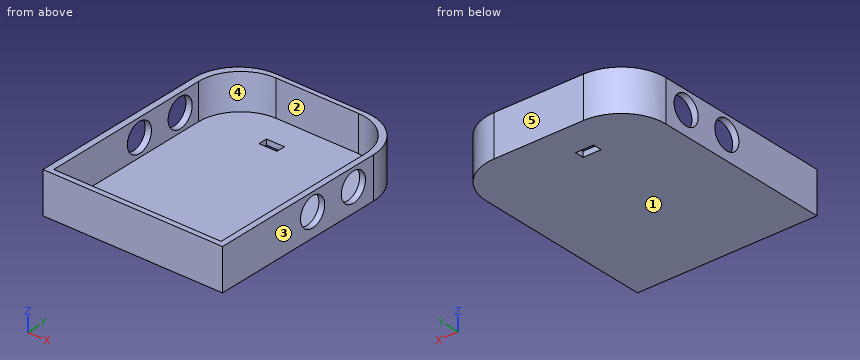
```python
from build123d import *

# Parameters (mm, degrees)
BOX008_W        = 10
BOX008_H        = 5
BOX008_DEPTH    = 10
PAD_DEPTH       = 23
POCKET_DEPTH    = 20
SKETCH002_R     = 8
POCKET001_DEPTH = 100.001


with BuildPart() as cube008:
    # Box008 → Box008 (new body)
    with BuildSketch(Plane(origin=(-15, 40, -4), x_dir=(1, 0, 0), z_dir=(0, 0, 1))):
        with Locations((5, 2.5)):
            Rectangle(BOX008_W, BOX008_H)
    extrude(amount=BOX008_DEPTH)


with BuildPart() as cut012:
    # Sketch → Pad (new body)
    with BuildSketch(Plane.XY):
        with BuildLine():
            Line((-50, 38.45712), (-50, -61.54288))
            Line((-50, -61.54288), (50, -61.54288))
            Line((50, -61.54288), (50, 38.45712))
            ThreePointArc((50, 38.45712), (42.67767, 56.13479), (25, 63.45712))
            Line((25, 63.45712), (-25, 63.45712))
            ThreePointArc((-25, 63.45712), (-42.67767, 56.13479), (-50, 38.45712))
        make_face()
    extrude(amount=PAD_DEPTH)

    # Sketch001 → Pocket (cut)
    with BuildSketch(Plane.XY.offset(23)):
        with BuildLine():
            Line((-46.504223, 37.299377), (-46.504223, -58.589802))
            Line((-46.504223, -58.589802), (46.756358, -58.589802))
            Line((46.756358, -58.589802), (46.756358, 36.931984))
            ThreePointArc((46.756358, 36.931984), (39.747359, 53.853203), (22.82614, 60.862202))
            Line((22.82614, 60.862202), (-22.941398, 60.862202))
            ThreePointArc((-22.941398, 60.862202), (-39.602831, 53.96081), (-46.504223, 37.299377))
        make_face()
    extrude(amount=-POCKET_DEPTH, mode=Mode.SUBTRACT)

    # Sketch002 → Pocket001 (cut, through all)
    with BuildSketch(Plane.YZ.offset(50)):
        with Locations((-1.771652, 13)):
            Circle(SKETCH002_R)
        with Locations((25.228348, 13)):
            Circle(SKETCH002_R)
    extrude(amount=-POCKET001_DEPTH, mode=Mode.SUBTRACT)

    # Cut012: cut Cube008
    add(cube008.part, mode=Mode.SUBTRACT)


solid = cut012.part
```
Work out the finished part from the listing and answer in its coordinate system (mm). Face numbers are marked on the shaded views. A direction names the side the tool comes from. Coordinates: 2 decimals unless noted, no trailing zeros. Loops run counter-clockwise (first coordinate to the right, second up) from the corner with the lowest first, then second, coordinate; pieces in that order, holes last.
1) For the marked faces 4 and 5, determine the directions among +Z, -Z, +X, -X, +Y, -Y from which every point of the face is accessible in a straight line to the end or side of a thin tool.
Results:
face 4: +Z
face 5: +Z, -Z, +X, -X, +Y
2) Flat-ended cylindrical pins translate along their axes: pin 1 (0.9 mm diameter, centred on y = 42.5, z = 1.5, fed in from -X); pin 2 (13 mm diameter, centred on y = 25.23, z = 13, fed in from -X); pin 3 (2.5 mm diameter, centred on y = 42, z = 1, fed in from +X). Find the tip coordinate at first contact, or state that the pin passes through.
Results:
pin 1: stops at x = -49.74
pin 2: passes through
pin 3: stops at x = 49.89
3) Section A-A (z = 13) is taken. Give the vertices of the cut face in (x, y).
Results:
outline: (-50, -61.54) - (50, -61.54) - (50, -9.77) - (46.76, -9.77) - (46.76, -58.59) - (-46.5, -58.59) - (-46.5, -9.77) - (-50, -9.77) - close; (-50, 6.23) - (-46.5, 6.23) - (-46.5, 17.23) - (-50, 17.23) - close; (-50, 33.23) - (-46.5, 33.23) - (-46.5, 37.3) arc R23.56 cw to (-22.94, 60.86) - (22.83, 60.86) arc R23.93 cw to (46.76, 36.93) - (46.76, 33.23) - (50, 33.23) - (50, 38.46) arc R25 ccw to (25, 63.46) - (-25, 63.46) arc R25 ccw to (-50, 38.46) - close; (46.76, 6.23) - (50, 6.23) - (50, 17.23) - (46.76, 17.23) - close
4) Section C-C (x = 3.5) is taken. Give the vertices of the cut face in (y, z), plus the area to 3 significant figures.
Results:
outline: (-61.54, 0) - (63.46, 0) - (63.46, 23) - (60.86, 23) - (60.86, 3) - (-58.59, 3) - (-58.59, 23) - (-61.54, 23) - close
area: 486 mm2
5) For a pull along X with two mould halves and no side action, classify the marked faces 1, 2 and 3 as +X half, -X half, draft (parallel to the pull), parting line (faces both ways), or undercut.
Results:
face 1: draft
face 2: undercut
face 3: +X half
6) Consider probe 1 along X at (y, z) = (-10, 20.25); probe 2 along Y at (x, z) = (-5, 20.5); probe 3 along Z at (x, y) = (9, 57). Determine where each line is inside the solid, lowest interval first.
Results:
probe 1: x = -50 to -46.5, 46.76 to 50
probe 2: y = -61.54 to -58.59, 60.86 to 63.46
probe 3: z = 0 to 3
7) Section B-B (y = -42.5) is taken. Give the vertices of the cut face in (x, z), plus the area to 3 significant figures.
Results:
outline: (-50, 0) - (50, 0) - (50, 23) - (46.76, 23) - (46.76, 3) - (-46.5, 3) - (-46.5, 23) - (-50, 23) - close
area: 435 mm2
8) Section D-D (y = 24) is taken. Give the vertices of the cut face in (x, z).
Results:
outline: (-50, 0) - (50, 0) - (50, 5.09) - (46.76, 5.09) - (46.76, 3) - (-46.5, 3) - (-46.5, 5.09) - (-50, 5.09) - close; (-50, 20.91) - (-46.5, 20.91) - (-46.5, 23) - (-50, 23) - close; (46.76, 20.91) - (50, 20.91) - (50, 23) - (46.76, 23) - close
